from build123d import *

# Parameters (mm, degrees)
SKETCH1_W           = 240
SKETCH1_H           = 150
BOSS_EXTRUDE1_DEPTH = 25
SKETCH2_R           = 15
SKETCH2_R_2         = 22.5
CUT_EXTRUDE1_DEPTH  = 10
SKETCH3_R           = 15
CUT_EXTRUDE2_DEPTH  = 143.302494708


with BuildPart() as part:
    # Sketch1 → Boss-Extrude1 (new body)
    with BuildSketch(Plane.XY):
        Rectangle(SKETCH1_W, SKETCH1_H)
    extrude(amount=BOSS_EXTRUDE1_DEPTH)

    # Sketch2 → Cut-Extrude1 (cut)
    # profile 1 of 4: a face of its own
    with BuildSketch(Plane.XY.offset(25)):
        with Locations((10, 45)):
            Circle(SKETCH2_R)
    # profile 2 of 4: a face of its own
    with BuildSketch(Plane.XY.offset(25)):
        with Locations((80, 45)):
            Circle(SKETCH2_R)
    # profile 3 of 4: a face of its own
    with BuildSketch(Plane.XY.offset(25)):
        with BuildLine():
            Line((-105, -30), (-105, 40))
            ThreePointArc((-105, 40), (-85, 60), (-65, 40))
            Line((-65, 40), (-65, -30))
            ThreePointArc((-65, -30), (-85, -50), (-105, -30))
        make_face()
    # profile 4 of 4: a face of its own
    with BuildSketch(Plane.XY.offset(25)):
        with BuildLine():
            Line((15, 15), (120, 15))
            Line((120, 15), (120, -75))
            Line((120, -75), (-30, -75))
            Line((-30, -75), (-30, -30))
            ThreePointArc((-30, -30), (-16.819805153, 1.819805153), (15, 15))
        make_face()
        with Locations((15, -30)):
            Circle(SKETCH2_R_2, mode=Mode.SUBTRACT)
    extrude(amount=-CUT_EXTRUDE1_DEPTH, mode=Mode.SUBTRACT)

    # Sketch3 → Cut-Extrude2 (cut, through all)
    with BuildSketch(Plane.XY.offset(15)):
        with Locations((10, 45)):
            Circle(SKETCH3_R)
        with Locations((80, 45)):
            Circle(SKETCH3_R)
    extrude(amount=-CUT_EXTRUDE2_DEPTH, mode=Mode.SUBTRACT)


solid = part.part
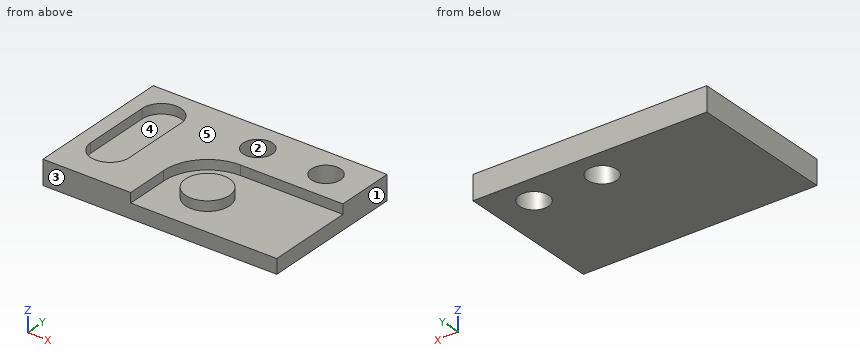
Input: part model. Units: mm. Frame: model coordinates. Face numbers are marked on the shaded views. A direction names the side the tool comes from. Coordinates: 2 decimals unless noted, no trailing zeros. Loops run counter-clockwise (first coordinate to the right, second up) from the corner with the lowest first, then second, coordinate; pieces in that order, holes last.
(1) Section C-C on x = -85. Return the cut outline in (y, z), then the cut area to 3 significant figures.
(2) Section A-A on z = 22.25. Return the cut outline in (x, y), then the cut area to 3 significant figures.
(3) Section B-B on x = 80. Return the cut outline in (y, z).
(4) Section D-D on y = 45. Return the cut outline in (x, z).
(5) Material intervals for probe 1 along Y at (x, z) = (80, 19.25); probe 2 along Y at (x, z) = (80, 10.25); probe 3 along X at (y, z) = (47, 20.5) (3 decimals), sorted ascending.
(6) First-contact query: pin 1 Ø5 at (x, z) = (51.5, 21.5) entering from -Y; pin 2 Ø12 at (x, y) = (-82, 13) entering from +Z; pin 3 Ø3 at (y, z) = (7.5, 20.5) entering from +X. Flat tips, straight axial feed; report the tip coordinate or a pass-through.
(7) Set-up query: the marked faces 4 and 5. Return all of +Z, -Z, +X, -X, +Y, -Y with unobstructed straight access to the full face (end or side cutting, diameter ignored); none if empty.
(8) Pull-direction query (X, two-part tool) for the marked faces 1, 2 and 3; classes: released by +X, released by -X, zero draft, split by the parting line, or undercut.
Data:
1. outline: (-75, 0) - (75, 0) - (75, 25) - (60, 25) - (60, 15) - (-50, 15) - (-50, 25) - (-75, 25) - close
1. area: 2,650 mm2
2. outline: (-120, -75) - (-30, -75) - (-30, -30) arc R45 cw to (15, 15) - (120, 15) - (120, 75) - (-120, 75) - close; circle Ø45 at (15, -30); hole (-105, -30) arc R20 ccw to (-65, -30) - (-65, 40) arc R20 ccw to (-105, 40) - close; hole circle Ø30 at (10, 45); hole circle Ø30 at (80, 45)
2. area: 19,100 mm2
3. outline: (-75, 0) - (30, 0) - (30, 25) - (15, 25) - (15, 15) - (-75, 15) - close; (60, 0) - (75, 0) - (75, 25) - (60, 25) - close
4. outline: (-120, 0) - (-5, 0) - (-5, 25) - (-65.64, 25) - (-65.64, 15) - (-104.36, 15) - (-104.36, 25) - (-120, 25) - close; (25, 0) - (65, 0) - (65, 25) - (25, 25) - close; (95, 0) - (120, 0) - (120, 25) - (95, 25) - close
5. probe 1: y = 15 to 30, 60 to 75
5. probe 2: y = -75 to 30, 60 to 75
5. probe 3: x = -120 to -103.735, -66.265 to -4.866, 24.866 to 65.134, 94.866 to 120
6. pin 1: stops at y = 15
6. pin 2: stops at z = 15
6. pin 3: stops at x = -7.45
7. face 4: +Z
7. face 5: +Z, +X, -X, +Y, -Y
8. face 1: released by +X
8. face 2: undercut
8. face 3: zero draft
